Verification items for the finished model (mm, model axes). A direction names the side the tool comes from. Round coordinates to 2 decimals unless told otherwise and drop trailing zeros. Order: outer loops, then holes, each group sorted by start corner. A loop starts at its lowest first (then second) coordinate and runs counter-clockwise, first axis right, second up.
```python
from build123d import *

# Parameters (mm, degrees)
EXTRUDE_1_DEPTH     = 13.9
SKETCH_2_R          = 1.25
CUT_EXTRUDE_1_DEPTH = 38.552762881


with BuildPart() as part:
    # 草图1 → 凸台-拉伸1 (new body)
    with BuildSketch(Plane(origin=(0, 0, 0), x_dir=(1, 0, 0), z_dir=(0, 1, 0))):
        with BuildLine():
            Line((0, 0), (15.912485012, 0))
            Line((15.912485012, 0), (15.912485012, 4.4))
            ThreePointArc((15.912485012, 4.4), (13.226409808, 4.729902507), (10.7, 5.7))
            Line((10.7, 5.7), (3.9, 5.7))
            Line((3.9, 5.7), (3.9, 8.3))
            Line((3.9, 8.3), (7.464408308, 8.3))
            ThreePointArc((7.464408308, 8.3), (4.812485012, 15.5), (7.464408308, 22.7))
            Line((7.464408308, 22.7), (3.9, 22.7))
            Line((3.9, 22.7), (3.9, 25.3))
            Line((3.9, 25.3), (10.7, 25.3))
            ThreePointArc((10.7, 25.3), (13.26888799, 26.28060271), (16, 26.599655))
            Line((16, 26.599655), (16, 31))
            Line((16, 31), (0, 31))
            Line((0, 31), (0, 0))
        make_face()
    extrude(amount=EXTRUDE_1_DEPTH)

    # 草图2 → 切除-拉伸1 (cut, through all)
    with BuildSketch(Plane.ZY):
        with Locations((-28.75, 10.95)):
            Circle(SKETCH_2_R)
        with Locations((-2.25, 10.95)):
            Circle(SKETCH_2_R)
        with Locations((-2.25, 2.95)):
            Circle(SKETCH_2_R)
        with Locations((-28.75, 2.95)):
            Circle(SKETCH_2_R)
    extrude(amount=-CUT_EXTRUDE_1_DEPTH, mode=Mode.SUBTRACT)


solid = part.part
```
1) Sectioned sample at D-D on x = 2.5. Record the cut outline in (y, z).
2) Draft check along Y on faces 4 (the cylindrical face through (7.888, 12.004, -28.078)), 5 (the flat face through (6, 7, -8.3)), 6 (the cylindrical face through (7.888, 2.471, -27.595)), 7 (the flat face through (4, 0, -16)). Enter one of: released by +Y, released by -Y, zero draft, split by the parting line, or undercut.
3) Scan lines: probe 1 along Y at (x, z) = (11.25, -2.25); probe 2 along Z at (x, y) = (6, 5.75); probe 3 along Z at (x, y) = (7.75, 9). Record each from-to range of solid material in increasing order.
4) Go/stop test with flat-tipped pins: pin 1 Ø3 at (y, z) = (2.95, -28.75) entering from +X; pin 2 Ø3.5 at (y, z) = (8, -1.5) entering from +X; pin 3 Ø1.3 at (y, z) = (6, -6.5) entering from +X; pin 4 Ø4 at (y, z) = (5, -20) entering from +X. Record where each tip stops, or that it passes through.
5) Tool access check on faces 1 (the flat face through (3.9, 7, -24)), 2 (the flat face through (0, 7, -16)), 3 (the flat face through (15.912, 7, -2)). Record the directions out of +Z, -Z, +X, -X, +Y, -Y that give a thin tool (end or side, any length) a straight path to the whole face; none if there is none.
6) Sectioned sample at A-A on x = 9.25. Record the cut outline in (y, z), then the cut area to 3 significant figures.
7) Sectioned sample at C-C on z = -28.75. Record the cut outline in (x, y), then the cut area to 3 significant figures.
8) Sectioned sample at B-B on y = 2.95. Record the cut outline in (x, z), then the cut area to 3 significant figures.
Returned:
1. outline: (0, -31) - (13.9, -31) - (13.9, 0) - (0, 0) - close; hole circle Ø2.5 at (2.95, -28.75); hole circle Ø2.5 at (2.95, -2.25); hole circle Ø2.5 at (10.95, -28.75); hole circle Ø2.5 at (10.95, -2.25)
2. face 4: undercut
2. face 5: zero draft
2. face 6: undercut
2. face 7: released by -Y
3. probe 1: y = 0 to 1.7, 4.2 to 9.7, 12.2 to 13.9
3. probe 2: z = -31 to -25.3, -22.7 to -20.5, -10.5 to -8.3, -5.7 to 0
3. probe 3: z = -31 to -25.3, -5.7 to 0
4. pin 1: stops at x = 16
4. pin 2: stops at x = 15.91
4. pin 3: stops at x = 3.9
4. pin 4: stops at x = 6.91
5. face 1: +X, +Y, -Y
5. face 2: +Z, -Z, -X, +Y, -Y
5. face 3: +Z, +X, +Y, -Y
6. outline: (0, -31) - (13.9, -31) - (13.9, -25.3) - (0, -25.3) - close; (0, -5.7) - (13.9, -5.7) - (13.9, 0) - (0, 0) - close; hole circle Ø2.5 at (2.95, -28.75); hole circle Ø2.5 at (2.95, -2.25); hole circle Ø2.5 at (10.95, -28.75); hole circle Ø2.5 at (10.95, -2.25)
6. area: 139 mm2
7. outline: (0, 0) - (16, 0) - (16, 1.7) - (0, 1.7) - close; (0, 4.2) - (16, 4.2) - (16, 9.7) - (0, 9.7) - close; (0, 12.2) - (16, 12.2) - (16, 13.9) - (0, 13.9) - close
7. area: 142 mm2
8. outline: (0, -31) - (16, -31) - (16, -30) - (0, -30) - close; (0, -27.5) - (16, -27.5) - (16, -26.6) arc R11.1 cw to (10.7, -25.3) - (3.9, -25.3) - (3.9, -22.7) - (7.46, -22.7) arc R11.1 cw to (7.46, -8.3) - (3.9, -8.3) - (3.9, -5.7) - (10.7, -5.7) arc R11.1 cw to (15.91, -4.4) - (15.91, -3.5) - (0, -3.5) - close; (0, -1) - (15.91, -1) - (15.91, 0) - (0, 0) - close
8. area: 194 mm2
